Source: CAD feature listing. Evaluate the final solid. Frame: model axes, mm. A direction names the side the tool comes from. Coordinates: 2 decimals unless noted, no trailing zeros. Order: outer loops, then holes, each group sorted by start corner. A loop starts at its lowest first (then second) coordinate and runs counter-clockwise, first axis right, second up. Notation, with made-up numbers: (-20, 79.25) -> (27, 79.25) arc R16 ccw to (27, 110.25) -> close; hole circle Ø10 at (36.25, -22.5). An arc over 180 degrees is marked (long way). Put each result on its own line as item: value.
from build123d import *

# Parameters (mm, degrees)
F0_R     = 7.5
F1_DEPTH = 3
F2_SIZE2 = 2.99999
F2_SIZE  = 1.99999
F3_R     = 2.4
F4_DEPTH = 5
F5_R     = 1


# Not quite as in the source:
# - a fillet or chamfer is up to 0.001 mm smaller than in the source, because OpenCascade refuses the exact size


with BuildPart() as f1:
    # F0 (on Top) → F1 (new body)
    with BuildSketch(Plane.XY):
        Circle(F0_R)
    extrude(amount=F1_DEPTH)

    # F2 (size 2 and 3 in the source; OpenCascade refuses exactly that, so slightly less here)
    f2_edges = [f1.edges().sort_by_distance(p)[0] for p in [
        (-7.5, 0, 3),
    ]]
    f2_side = f1.faces().sort_by_distance((0, 0, 3))[0]
    chamfer(f2_edges, length=F2_SIZE, length2=F2_SIZE2, reference=f2_side)

    # F3 (on face) → F4 (join)
    with BuildSketch(Plane.XY.offset(3)):
        Circle(F3_R)
    extrude(amount=F4_DEPTH)

    # F5
    f5_edges = [f1.edges().sort_by_distance(p)[0] for p in [
        (-2.4, 0, 8),
        (-2.4, 0, 3),
    ]]
    fillet(f5_edges, radius=F5_R)


solid = f1.part
1. Cut plane C-C on z = 6.75. Output: boundary loops of the cut face in (x, y).
Numbers:
outline: circle Ø4.8 at (0, 0)
2. Cut plane D-D on z = 2.25. Output: boundary loops of the cut face in (x, y), plus the area to 3 significant figures.
Numbers:
outline: circle Ø12 at (0, 0)
area: 113 mm2
3. Ray query, line 1 along Z through (x, y) = (-0.25, -4.5); line 2 along X through (y, z) = (-3.75, 1.25); line 3 along X through (y, z) = (0.5, 3.5). Return the intervals inside material, ascending.
Numbers:
line 1: z = 0 to 3
line 2: x = -5.51 to 5.51
line 3: x = -2.48 to 2.48
4. Set-up query: faces 1 (the flat face through (2, 3, 3)), 2 (the flat face through (0, 0, 0)). Return all of +Z, -Z, +X, -X, +Y, -Y with unobstructed straight access to the full face (end or side cutting, diameter ignored); none if empty.
Numbers:
face 1: +Z
face 2: -Z, +X, -X, +Y, -Y
5. First-contact query: pin 1 (2 mm diameter, centred on y = 0, z = 5.5, fed in from -X); pin 2 (1 mm diameter, centred on x = -5, z = 2.5, fed in from -Y). Flat tips, straight axial feed; report the tip coordinate or a pass-through.
Numbers:
pin 1: stops at x = -2.4
pin 2: stops at y = -3.91
